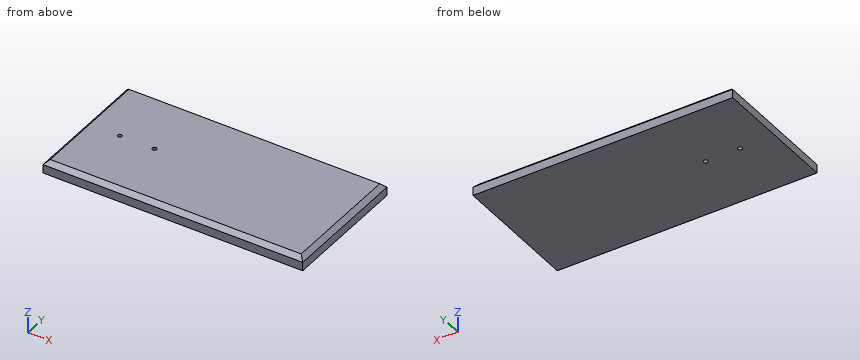
```python
from build123d import *

# Parameters (mm, degrees)
F0_W     = 300
F0_H     = 150
F1_DEPTH = 15
F2_SIZE  = 5.08
F4_D     = 5


with BuildPart() as f1:
    # F0 (on Top) → F1 (new body)
    with BuildSketch(Plane.XY):
        with Locations((150, 75)):
            Rectangle(F0_W, F0_H)
    extrude(amount=F1_DEPTH)

    # F2
    f2_edges = [f1.edges().sort_by_distance(p)[0] for p in [
        (150, 0, 15),
        (300, 75, 15),
        (150, 150, 15),
        (0, 75, 15),
    ]]
    chamfer(f2_edges, length=F2_SIZE)

    # F4 (through all)
    with Locations(Plane(origin=(0, 0, 0), x_dir=(1, 0, 0), z_dir=(0, 0, -1))):
        with Locations((40, -75), (80, -75)):
            Hole(F4_D / 2)


solid = f1.part
```
Geometry check sheet. Reference: the model listing, model coordinates, mm. Round coordinates to 2 decimals unless told otherwise and drop trailing zeros. Order: outer loops, then holes, each group sorted by start corner. A loop starts at its lowest first (then second) coordinate and runs counter-clockwise, first axis right, second up. Notation, with made-up numbers: M 14.25,8.25 L 58.25,8.25 A18 ccw 58.25,12.25 Z; hole C 79.5,42.5 d6. An arc over 180 degrees is marked long. Write item = value, one per line.
Q1. Depth check by flat-ended pin: pin 1 Ø1.5 at (x, z) = (169, 12.5) entering from +Y; pin 2 Ø6 at (x, y) = (80, 75) entering from -Z; pin 3 Ø1 at (x, z) = (116.5, 10.5) entering from -Y; pin 4 Ø5 at (x, z) = (157, 12.5) entering from +Y. Enter the tip coordinate at first touch or a pass-through.
Answer block:
pin_1 = 148.17
pin_2 = 0
pin_3 = 0.08
pin_4 = 149.92
Q2. Section check A-A (z = 12.25). Enter the section's corners in (x, y), plus the area to 3 significant figures.
Answer block:
outline = M 2.33,2.33 L 297.67,2.33 L 297.67,147.67 L 2.33,147.67 Z; hole C 40,75 d5; hole C 80,75 d5
area = 42,900 mm^2
Q3. Scan lines: line 1 (X direction, y = 75, z = 5.25); line 2 (Y direction, x = 80, z = 4); line 3 (Y direction, x = 80, z = 11.5). Record each from-to range of solid material in increasing order.
Answer block:
line_1 = 0 to 37.5, 42.5 to 77.5, 82.5 to 300
line_2 = 0 to 72.5, 77.5 to 150
line_3 = 1.58 to 72.5, 77.5 to 148.42
